Read the model definition and answer for the solid it produces. Units are mm, in the model's axes. A direction names the side the tool comes from. Give positions to 0.01 mm unless a question says otherwise; leave off trailing zeros. Order: outer loops, then holes, each group sorted by start corner. A loop starts at its lowest first (then second) coordinate and runs counter-clockwise, first axis right, second up. Notation, with made-up numbers: (-2.75, 14.25) - (8.25, 14.25) arc R16 ccw to (8.25, 44.25) - close; hole circle Ø5 at (25, 56). An arc over 180 degrees is marked (long way). One line per item, written item: value. Start each with the question number.
```python
from build123d import *

# Parameters (mm, degrees)
F0_W      = 55
F0_H      = 10
F1_DEPTH  = 10
F3_D      = 2.8
F3_DEPTH  = 13
F3_TIP    = 0.8412048666
F5_D      = 2.8
F5_DEPTH  = 13
F5_TIP    = 0.8412048666
F7_DEPTH  = 2.5
F9_DEPTH  = 2.5
F10_R     = 4.9999
F12_D     = 1.8
F12_DEPTH = 5
F12_TIP   = 0.5407745571


# Not quite as in the source:
# - a fillet or chamfer is up to 0.001 mm smaller than in the source, because OpenCascade refuses the exact size
# - a feature names something its author has since deleted; it is built from what else it names


with BuildPart() as f1:
    # F0 (on Top) → F1 (new body)
    with BuildSketch(Plane.XY):
        Rectangle(F0_W, F0_H)
    extrude(amount=F1_DEPTH)

    # F3
    with Locations(Plane(origin=(-27.5, 0, 0), x_dir=(0, -1, 0), z_dir=(-1, 0, 0))):
        with Locations((0, 5)):
            Hole(F3_D / 2, depth=F3_DEPTH)
            with Locations((0, 0, -(F3_DEPTH + F3_TIP / 2))):  # 118° drill point
                Cone(0, F3_D / 2, F3_TIP, mode=Mode.SUBTRACT)

    # F5
    with Locations(Plane.YZ.offset(27.5)):
        with Locations((0, 5)):
            Hole(F5_D / 2, depth=F5_DEPTH)
            with Locations((0, 0, -(F5_DEPTH + F5_TIP / 2))):  # 118° drill point
                Cone(0, F5_D / 2, F5_TIP, mode=Mode.SUBTRACT)

    # F6 (on face) → F7 (cut)
    with BuildSketch(Plane.YZ.offset(27.5)):
        with BuildLine():
            Line((5, 0), (5, 5))
            ThreePointArc((5, 5), (3.5355339059, 1.4644660941), (0, 0))
            Line((0, 0), (5, 0))
        make_face()
        with BuildLine():
            Line((-5, 0), (0, 0))
            ThreePointArc((0, 0), (-3.5355339059, 1.4644660941), (-5, 5))
            Line((-5, 5), (-5, 0))
        make_face()
    extrude(amount=-F7_DEPTH, mode=Mode.SUBTRACT)

    # F8 (on face) → F9 (cut)
    with BuildSketch(Plane(origin=(-27.5, 0, 0), x_dir=(0, -1, 0), z_dir=(-1, 0, 0))):
        with BuildLine():
            Line((5, 0), (5, 5))
            ThreePointArc((5, 5), (3.5355339059, 1.4644660941), (0, 0))
            Line((0, 0), (5, 0))
        make_face()
        with BuildLine():
            ThreePointArc((0, 10), (3.5355339059, 8.5355339059), (5, 5))
            Line((5, 5), (5, 10))
            Line((5, 10), (0, 10))
        make_face()
        with BuildLine():
            Line((-5, 0), (0, 0))
            ThreePointArc((0, 0), (-3.5355339059, 1.4644660941), (-5, 5))
            Line((-5, 5), (-5, 0))
        make_face()
    extrude(amount=-F9_DEPTH, mode=Mode.SUBTRACT)

    # F10 (radius 5 in the source; OpenCascade refuses exactly that, so slightly less here)
    f10_edges = [f1.edges().sort_by_distance(p)[0] for p in [
        (0, 5, 10),
        (1.25, -5, 10),
    ]]
    fillet(f10_edges, radius=F10_R)

    # F12
    with Locations(Plane(origin=(0, 0, 0), x_dir=(1, 0, 0), z_dir=(0, 0, -1))):
        with Locations((-20, 0), (20, 0)):
            Hole(F12_D / 2, depth=F12_DEPTH)
            with Locations((0, 0, -(F12_DEPTH + F12_TIP / 2))):  # 118° drill point
                Cone(0, F12_D / 2, F12_TIP, mode=Mode.SUBTRACT)


solid = f1.part
```
1) The mould has two halves that part along Y. Classify faces 1 (the flat face through (1, -5, 2)), 2 (the flat face through (25, 4, 1)), 3 (the conical face through (13.805, -0.053, 4.763)): +Y half, -Y half, draft (parallel to the pull), parting line (faces both ways), or undercut.
2) For faces 4 (the flat face through (-25, -4, 1)), 5 (the flat face through (25, -4, 1)), 6 (the cylindrical face through (20.12, -0.89, 1.99)), 7 (the cylindrical face through (-20.91, -0.18, 6.39)), 8 (the cylindrical face through (20.91, 0.18, 6.39)), determine the directions among +Z, -Z, +X, -X, +Y, -Y from which every point of the face is accessible in a straight line to the end or side of a thin tool.
3) Each of these flat-tipped pins is pushed along its axis until it touches: pin 1 (3 mm diameter, centred on x = 10, z = 7.5, fed in from -Y); pin 2 (1.7 mm diameter, centred on y = 0, z = 5, fed in from -X); pin 3 (1.5 mm diameter, centred on x = -19.5, z = 5.5, fed in from -Y); pin 4 (2 mm diameter, centred on y = 0, z = 5, fed in from -X). Where does it stop, or does it pass through?
4) Find the intervals of material crossed by probe 1 along Y at (x, z) = (20, 2.15); probe 2 along Y at (x, z) = (-24.75, 5); probe 3 along Z at (x, y) = (-19.5, 0), in increasing order. Write a range as from..to.
5) Section A-A on z = 2 is taken. Write down the section's boundary in (x, y), plus the area to 3 significant figures.
Solved:
1. face 1: -Y half
1. face 2: draft
1. face 3: undercut
2. face 4: -Z, -X, -Y
2. face 5: -Z, +X, -Y
2. face 6: -Z
2. face 7: -X
2. face 8: +X
3. pin 1: stops at y = -4.9
3. pin 2: stops at x = -14.17
3. pin 3: stops at y = -5
3. pin 4: stops at x = -14.26
4. probe 1: y = -5..-0.9, 0.9..5
4. probe 2: y = -5..-1.4, 1.4..5
4. probe 3: z = 6.4..10
5. outline: (-27.5, -4) - (-25, -4) - (-25, -5) - (25, -5) - (25, -4) - (27.5, -4) - (27.5, 4) - (25, 4) - (25, 5) - (-25, 5) - (-25, 4) - (-27.5, 4) - close; hole circle Ø1.8 at (-20, 0); hole circle Ø1.8 at (20, 0)
5. area: 535 mm2
